The listing builds one solid part. Answer for the finished solid, in the listing's coordinates (mm). Face numbers are marked on the shaded views. A direction names the side the tool comes from. Give positions to 0.01 mm unless a question says otherwise; leave off trailing zeros. Write each loop counter-clockwise with the first axis right and the second up, starting at its lowest first coordinate (ties: lowest second). Pieces come first, ordered by that corner, then holes. Notation, with made-up numbers: (25, -30.75) - (43, -30.75) arc R29 ccw to (43, 3.25) - close; hole circle Ø2 at (-31.5, -20.5). An arc over 180 degrees is marked (long way). Answer in a Markdown table with one row per item. Add a question column.
from build123d import *

# Parameters (mm, degrees)
ESTRUSIONE_ESTRUSIONE1_DEPTH                         = 4
ESTRUSIONE_ESTRUSIONE1_2_DEPTH                       = 4
ESTRUSIONE_ESTRUSIONE2_DEPTH                         = 9
ESTRUSIONE_ESTRUSIONE3_DEPTH                         = 9
RACCORDO1_R                                          = 10
FORO_LAMATO_PER_VITE_M4_A_TESTA_CILINDRI_D           = 4.5
FORO_LAMATO_PER_VITE_M4_A_TESTA_CILINDRI_DEPTH       = 34
FORO_LAMATO_PER_VITE_M4_A_TESTA_CILINDRI_CBORE_D     = 10
FORO_LAMATO_PER_VITE_M4_A_TESTA_CILINDRI_CBORE_DEPTH = 2.6
FORO_LAMATO_PER_VITE_M4_A_TESTA_CILINDRI_TIP         = 1.351936393
FORO_PER_VITE_M4_1_D                                 = 4.2
FORO_PER_VITE_M4_1_DEPTH                             = 8
FORO_PER_VITE_M4_1_TIP                               = 1.2618073


with BuildPart() as part:
    # Schizzo3 → Estrusione-Estrusione1 (new body)
    with BuildSketch(Plane.XY):
        Polygon((-30, 10.25), (30, 10.25), (30, 14.25), (15, 14.25), (7.5, 25.25), (-7.5, 25.25), (-15, 14.25), (-30, 14.25), align=None)
    extrude(amount=ESTRUSIONE_ESTRUSIONE1_DEPTH)



with BuildPart() as body_2:
    # Schizzo3 → Estrusione-Estrusione1 2 (new body)
    with BuildSketch(Plane.XY):
        Polygon((30, -10.25), (-30, -10.25), (-30, -14.25), (-15, -14.25), (-7.5, -25.25), (7.5, -25.25), (15, -14.25), (30, -14.25), align=None)
    extrude(amount=ESTRUSIONE_ESTRUSIONE1_2_DEPTH)


with BuildPart() as part_1:
    add(part.part)

    add(body_2.part)  # Estrusione-Estrusione2 merges body 2
    # Schizzo4 → Estrusione-Estrusione2 (add)
    with BuildSketch(Plane.ZY.offset(30)):
        Polygon((18, 10.25), (4, 14.25), (4, 10.25), (8, 9.107142857), (8, -9.107142857), (4, -10.25), (4, -14.25), (18, -10.25), align=None)
    extrude(amount=-ESTRUSIONE_ESTRUSIONE2_DEPTH)

    # Schizzo5 → Estrusione-Estrusione3 (add)
    with BuildSketch(Plane(origin=(30, 0, 0), x_dir=(0, 0, -1), z_dir=(1, 0, 0))):
        Polygon((-4, -14.25), (-18, -10.25), (-18, 10.25), (-4, 14.25), (-4, 10.25), (-8, 9.107142857), (-8, -9.107142857), (-4, -10.25), align=None)
    extrude(amount=-ESTRUSIONE_ESTRUSIONE3_DEPTH)

    # Raccordo1
    raccordo1_edges = [part_1.edges().sort_by_distance(p)[0] for p in [
        (-7.5, 25.25, 2),
        (7.5, 25.25, 2),
        (-7.5, -25.25, 2),
        (7.5, -25.25, 2),
    ]]
    fillet(raccordo1_edges, radius=RACCORDO1_R)

    # Foro lamato per Vite M4 a testa cilindrica piana-1
    with Locations(Plane.XY.offset(4)):
        with Locations((0, 17.75), (0, -17.75)):
            CounterBoreHole(FORO_LAMATO_PER_VITE_M4_A_TESTA_CILINDRI_D / 2, FORO_LAMATO_PER_VITE_M4_A_TESTA_CILINDRI_CBORE_D / 2, FORO_LAMATO_PER_VITE_M4_A_TESTA_CILINDRI_CBORE_DEPTH, depth=FORO_LAMATO_PER_VITE_M4_A_TESTA_CILINDRI_DEPTH)
            with Locations((0, 0, -(FORO_LAMATO_PER_VITE_M4_A_TESTA_CILINDRI_DEPTH + FORO_LAMATO_PER_VITE_M4_A_TESTA_CILINDRI_TIP / 2))):  # 118° drill point
                Cone(0, FORO_LAMATO_PER_VITE_M4_A_TESTA_CILINDRI_D / 2, FORO_LAMATO_PER_VITE_M4_A_TESTA_CILINDRI_TIP, mode=Mode.SUBTRACT)

    # Foro per Vite M4-1
    with Locations(Plane.XY.offset(18)):
        with Locations((-26, -6.05), (25, 6.05), (25, -6.05), (-26, 6.05)):
            Hole(FORO_PER_VITE_M4_1_D / 2, depth=FORO_PER_VITE_M4_1_DEPTH)
            with Locations((0, 0, -(FORO_PER_VITE_M4_1_DEPTH + FORO_PER_VITE_M4_1_TIP / 2))):  # 118° drill point
                Cone(0, FORO_PER_VITE_M4_1_D / 2, FORO_PER_VITE_M4_1_TIP, mode=Mode.SUBTRACT)


solid = part_1.part
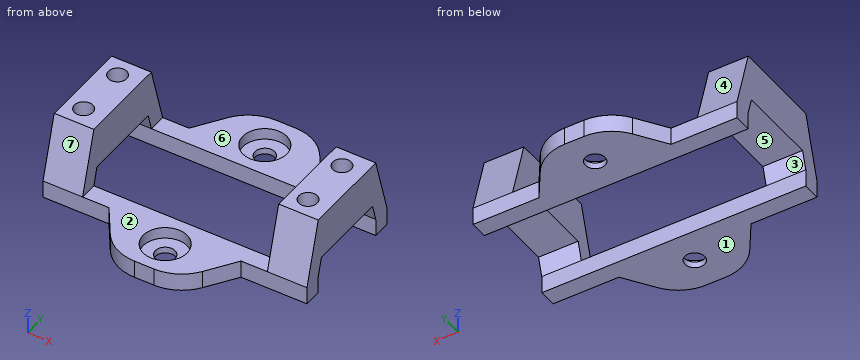
1. Section C-C (z = 14.25) is taken. Give the vertices of the cut face in (x, y), and give its area (3 significant figures).
2. Straight lines are drawn through the part: L1, parallel to X at y = 6.05, z = 16.5; L2, parallel to Y at x = 0, z = 0.3; L3, parallel to X at y = 11, z = 14. For each, find the intervals that lie inside material, in ascending order. Write a range as [from, to].
3. Section A-A (z = 3) is taken. Give the vertices of the cut face in (x, y), and give its area (3 significant figures).
4. Given pin 1 Ø4 at (x, z) = (23.5, 9) entering from +Y; pin 2 Ø1.2 at (x, z) = (-25.5, 2) entering from +Y; pin 3 Ø5 at (x, y) = (-1.5, 15.5) entering from +Z, each flat-ended and moving along its own axis, determine where each tip first touches the part or whether it passes through.
5. The mould has two halves that part along Y. Classify the marked faces 4, 5, 6 and 7: +Y half, -Y half, draft (parallel to the pull), parting line (faces both ways), or undercut.
6. A tool of negligible diameter and unlimited length cuts with its end or side. For the marked faces 1, 2 and 3, from which of +Z, -Z, +X, -X, +Y, -Y can it reach the whole face along a straight path? Write none if from no direction.
7. Section D-D (x = -23) is taken. Give the vertices of the cut face in (y, z).
8. Section B-B (x = 0) is taken. Give the vertices of the cut face in (y, z), and give its area (3 significant figures).
Geometry check:
| question | item | result |
|---|---|---|
| 1 | outline | (-30, -11.32) - (-21, -11.32) - (-21, 11.32) - (-30, 11.32) - close; (21, -11.32) - (30, -11.32) - (30, 11.32) - (21, 11.32) - close; hole circle Ø4.2 at (-26, -6.05); hole circle Ø4.2 at (-26, 6.05); hole circle Ø4.2 at (25, -6.05); hole circle Ø4.2 at (25, 6.05) |
| 1 | area | 352 mm² |
| 2 | L1 | [-30, -28.1], [-23.9, -21], [21, 22.9], [27.1, 30] |
| 2 | L2 | [-25.25, -20], [-15.5, -10.25], [10.25, 15.5], [20, 25.25] |
| 2 | L3 | [-30, -21], [21, 30] |
| 3 | outline | (-30, -14.25) - (-15, -14.25) - (-10.48, -20.88) arc R10 ccw to (-2.21, -25.25) - (2.21, -25.25) arc R10 ccw to (10.48, -20.88) - (15, -14.25) - (30, -14.25) - (30, -10.25) - (-30, -10.25) - close; (-30, 10.25) - (30, 10.25) - (30, 14.25) - (15, 14.25) - (10.48, 20.88) arc R10 ccw to (2.21, 25.25) - (-2.21, 25.25) arc R10 ccw to (-10.48, 20.88) - (-15, 14.25) - (-30, 14.25) - close; hole circle Ø10 at (0, -17.75); hole circle Ø10 at (0, 17.75) |
| 3 | area | 801 mm² |
| 4 | pin 1 | y = 13.39 |
| 4 | pin 2 | y = 14.25 |
| 4 | pin 3 | z = 4 |
| 5 | face 4 | +Y half |
| 5 | face 5 | undercut |
| 5 | face 6 | draft |
| 5 | face 7 | -Y half |
| 6 | face 1 | -Z, +X, -X, +Y, -Y |
| 6 | face 2 | +Z, +Y, -Y |
| 6 | face 3 | -Z, +X, -X |
| 7 | outline | (-14.25, 0) - (-10.25, 0) - (-10.25, 4) - (-9.11, 8) - (9.11, 8) - (10.25, 4) - (10.25, 0) - (14.25, 0) - (14.25, 4) - (10.25, 18) - (-10.25, 18) - (-14.25, 4) - close |
| 8 | outline | (-25.25, 0) - (-20, 0) - (-20, 1.4) - (-22.75, 1.4) - (-22.75, 4) - (-25.25, 4) - close; (-15.5, 0) - (-10.25, 0) - (-10.25, 4) - (-12.75, 4) - (-12.75, 1.4) - (-15.5, 1.4) - close; (10.25, 0) - (15.5, 0) - (15.5, 1.4) - (12.75, 1.4) - (12.75, 4) - (10.25, 4) - close; (20, 0) - (25.25, 0) - (25.25, 4) - (22.75, 4) - (22.75, 1.4) - (20, 1.4) - close |
| 8 | area | 55.4 mm² |
